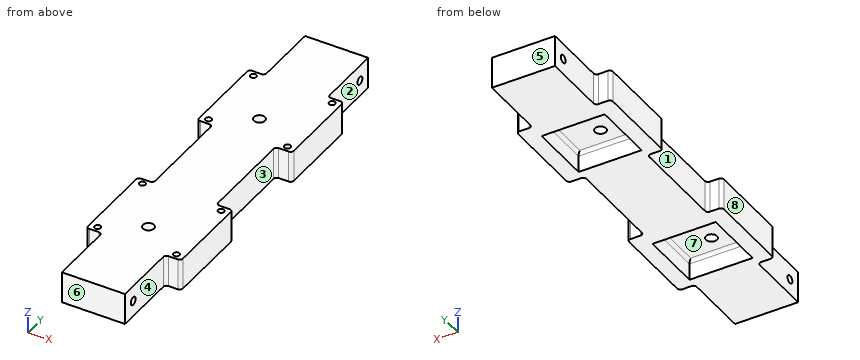
```python
from build123d import *

# Parameters (mm, degrees)
SKETCH1_W                        = 69.85
SKETCH1_H                        = 76.2
SKETCH1_R                        = 4.445
BOSS_EXTRUDE1_DEPTH              = 25.4
SKETCH2_W                        = 50.8
SKETCH2_H                        = 49.911
CUT_EXTRUDE1_DEPTH               = 15.875
SKETCH4_W                        = 50.8
SKETCH4_H                        = 25.4
BOSS_EXTRUDE2_DEPTH              = 79.9846
SKETCH7_W                        = 76.2
SKETCH7_H                        = 25.4
BOSS_EXTRUDE5_DEPTH              = 69.85
SKETCH10_R                       = 4.445
CUT_EXTRUDE3_DEPTH               = 191.349362468
SKETCH11_W                       = 50.8
SKETCH11_H                       = 49.911
CUT_EXTRUDE4_DEPTH               = 15.875
SKETCH12_W                       = 50.8
SKETCH12_H                       = 25.4
BOSS_EXTRUDE7_DEPTH              = 54.4576
SKETCH13_W                       = 50.8
SKETCH13_H                       = 25.4
BOSS_EXTRUDE8_DEPTH              = 54.2798
F_10_0_1935_DIAMETER_HOLE2_D     = 4.9149
F_10_0_1935_DIAMETER_HOLE2_DEPTH = 11.938
F_10_0_1935_DIAMETER_HOLE2_TIP   = 1.476584928
SKETCH18_R                       = 3.2639
CUT_EXTRUDE5_DEPTH               = 12.7
CUT_EXTRUDE6_START               = -12.7
SKETCH19_R                       = 3.2639
CUT_EXTRUDE6_DEPTH               = 12.7
SKETCH20_R                       = 3.2639
CUT_EXTRUDE7_DEPTH               = 12.7
CUT_EXTRUDE8_START               = -12.7
SKETCH21_R                       = 3.2639
CUT_EXTRUDE8_DEPTH               = 12.7
F_10_0_1935_DIAMETER_HOLE3_D     = 4.9149
F_10_0_1935_DIAMETER_HOLE3_DEPTH = 11.938
F_10_0_1935_DIAMETER_HOLE3_TIP   = 1.476584928
FILLET1_R                        = 2.54
FILLET2_R                        = 2.54


with BuildPart() as part:
    # Sketch1 → Boss-Extrude1 (new body)
    with BuildSketch(Plane(origin=(0, 0, 0), x_dir=(0, 1, 0), z_dir=(0, 0, 1))):
        Rectangle(SKETCH1_W, SKETCH1_H)
        with Locations(Location((-11.811, 1.778, 0), (0, 0, 270))):
            Circle(SKETCH1_R, mode=Mode.SUBTRACT)
    extrude(amount=BOSS_EXTRUDE1_DEPTH)

    # Sketch2 → Cut-Extrude1 (cut)
    with BuildSketch(Plane(origin=(0, 0, 0), x_dir=(1, 0, 0), z_dir=(0, 0, -1))):
        with Locations((0, 2.7305)):
            Rectangle(SKETCH2_W, SKETCH2_H)
    extrude(amount=-CUT_EXTRUDE1_DEPTH, mode=Mode.SUBTRACT)

    # Sketch4 → Boss-Extrude2 (add)
    with BuildSketch(Plane(origin=(0, 34.925, 0), x_dir=(-1, 0, 0), z_dir=(0, 1, 0))):
        with Locations((0.465931196, 12.7)):
            Rectangle(SKETCH4_W, SKETCH4_H)
    extrude(amount=BOSS_EXTRUDE2_DEPTH)

    # Sketch7 → Boss-Extrude5 (add)
    with BuildSketch(Plane(origin=(0, 114.9096, 0), x_dir=(-1, 0, 0), z_dir=(0, 1, 0))):
        with Locations((0, 12.7)):
            Rectangle(SKETCH7_W, SKETCH7_H)
    extrude(amount=BOSS_EXTRUDE5_DEPTH)

    # Sketch10 → Cut-Extrude3 (cut, through all)
    with BuildSketch(Plane.XY.offset(25.4)):
        with Locations((-1.778, 138.0236)):
            Circle(SKETCH10_R)
    extrude(amount=-CUT_EXTRUDE3_DEPTH, mode=Mode.SUBTRACT)

    # Sketch11 → Cut-Extrude4 (cut)
    with BuildSketch(Plane(origin=(0, 0, 0), x_dir=(1, 0, 0), z_dir=(0, 0, -1))):
        with Locations((0, -147.1041)):
            Rectangle(SKETCH11_W, SKETCH11_H)
    extrude(amount=-CUT_EXTRUDE4_DEPTH, mode=Mode.SUBTRACT)

    # Sketch12 → Boss-Extrude7 (add)
    with BuildSketch(Plane(origin=(0, 184.7596, 0), x_dir=(-1, 0, 0), z_dir=(0, 1, 0))):
        with Locations((0, 12.7)):
            Rectangle(SKETCH12_W, SKETCH12_H)
    extrude(amount=BOSS_EXTRUDE7_DEPTH)

    # Sketch13 → Boss-Extrude8 (add)
    with BuildSketch(Plane.XZ.offset(34.925)):
        with Locations((0, 12.7)):
            Rectangle(SKETCH13_W, SKETCH13_H)
    extrude(amount=BOSS_EXTRUDE8_DEPTH)

    # #10 (0.1935) Diameter Hole2
    with Locations(Plane.XY.offset(25.4)):
        with Locations((31.75, 119.6721), (31.75, 179.9971), (-31.75, 179.9971), (-31.75, 119.6721)):
            Hole(F_10_0_1935_DIAMETER_HOLE2_D / 2, depth=F_10_0_1935_DIAMETER_HOLE2_DEPTH)
            with Locations((0, 0, -(F_10_0_1935_DIAMETER_HOLE2_DEPTH + F_10_0_1935_DIAMETER_HOLE2_TIP / 2))):  # 118° drill point
                Cone(0, F_10_0_1935_DIAMETER_HOLE2_D / 2, F_10_0_1935_DIAMETER_HOLE2_TIP, mode=Mode.SUBTRACT)

    # Sketch18 → Cut-Extrude5 (cut)
    with BuildSketch(Plane.YZ.offset(25.4)):
        with Locations(Location((228.1047, 12.7, 0), (0, 0, 270))):
            Circle(SKETCH18_R)
    extrude(amount=-CUT_EXTRUDE5_DEPTH, mode=Mode.SUBTRACT)

    # Sketch19 → Cut-Extrude6 (cut)
    with BuildSketch(Plane(origin=(-25.4, 0, 0), x_dir=(0, -1, 0), z_dir=(-1, 0, 0)).offset(CUT_EXTRUDE6_START)):
        with Locations(Location((-228.1047, 12.7, 0), (0, 0, 270))):
            Circle(SKETCH19_R)
    extrude(amount=CUT_EXTRUDE6_DEPTH, mode=Mode.SUBTRACT)

    # Sketch20 → Cut-Extrude7 (cut)
    with BuildSketch(Plane(origin=(-25.4, 0, 0), x_dir=(0, -1, 0), z_dir=(-1, 0, 0))):
        with Locations(Location((78.0923, 12.7, 0), (0, 0, 90))):
            Circle(SKETCH20_R)
    extrude(amount=-CUT_EXTRUDE7_DEPTH, mode=Mode.SUBTRACT)

    # Sketch21 → Cut-Extrude8 (cut)
    with BuildSketch(Plane.YZ.offset(25.4).offset(CUT_EXTRUDE8_START)):
        with Locations(Location((-78.0923, 12.7, 0), (0, 0, 90))):
            Circle(SKETCH21_R)
    extrude(amount=CUT_EXTRUDE8_DEPTH, mode=Mode.SUBTRACT)

    # #10 (0.1935) Diameter Hole3
    with Locations(Plane.XY.offset(25.4)):
        with Locations((31.75, -30.1625), (31.663484949, 30.1625), (-31.75, 30.1625), (-31.75, -30.1625)):
            Hole(F_10_0_1935_DIAMETER_HOLE3_D / 2, depth=F_10_0_1935_DIAMETER_HOLE3_DEPTH)
            with Locations((0, 0, -(F_10_0_1935_DIAMETER_HOLE3_DEPTH + F_10_0_1935_DIAMETER_HOLE3_TIP / 2))):  # 118° drill point
                Cone(0, F_10_0_1935_DIAMETER_HOLE3_D / 2, F_10_0_1935_DIAMETER_HOLE3_TIP, mode=Mode.SUBTRACT)

    # Fillet1
    fillet1_edges = [part.edges().sort_by_distance(p)[0] for p in [
        (-25.4, -34.925, 12.7),
        (25.4, -34.925, 12.7),
        (24.934068804, 34.925, 12.7),
        (-25.865931196, 34.925, 12.7),
        (24.934068804, 114.9096, 12.7),
        (-25.865931196, 114.9096, 12.7),
        (38.1, 114.9096, 12.7),
        (-38.1, 114.9096, 12.7),
        (38.1, 184.7596, 12.7),
        (-38.1, 184.7596, 12.7),
        (38.1, 34.925, 12.7),
        (38.1, -34.925, 12.7),
        (-38.1, -34.925, 12.7),
        (-38.1, 34.925, 12.7),
        (25.4, 184.7596, 12.7),
        (-25.4, 184.7596, 12.7),
    ]]
    fillet(fillet1_edges, radius=FILLET1_R)

    # Fillet2
    fillet2_edges = [part.edges().sort_by_distance(p)[0] for p in [
        (-25.4, -2.7305, 15.875),
        (0, -27.686, 15.875),
        (25.4, -2.7305, 15.875),
        (0, 22.225, 15.875),
        (-25.4, 147.1041, 15.875),
        (0, 122.1486, 15.875),
        (25.4, 147.1041, 15.875),
        (0, 172.0596, 15.875),
    ]]
    fillet(fillet2_edges, radius=FILLET2_R)


solid = part.part
```
Model file for the job. Use its own axes, mm. Face numbers are marked on the shaded views. A direction names the side the tool comes from. Round coordinates to 2 decimals unless told otherwise and drop trailing zeros. Loops run counter-clockwise (first coordinate to the right, second up) from the corner with the lowest first, then second, coordinate; pieces in that order, holes last. Notation, with made-up numbers: M 13,61 L 39,61 A30 ccw 39,86 Z; hole C 58.5,11 d2. An arc over 180 degrees is marked long. Put each result on its own line as item: value. Start each with the question number.
Item 1: Mould opens along Y. For the marked faces 5, 6, 7 and 8 say: released by +Y, released by -Y, zero draft, split by the parting line, or undercut.
Item 2: Cut at A-A (y = 6). List the corners of the cut face in (x, z) (3 decimals), then the cut area to 3 significant figures.
Item 3: Drop flat-ended pins along their axis: P1, Ø10, axis at x = -1.78, y = 138.02, coming from the -Z side (3 decimals); P2, Ø2, axis at y = -77, z = 11.5, coming from the +X side; P3, Ø6, axis at x = 33, z = 7.5, coming from the -Y side (3 decimals). Give the stop position or say it passes through.
Item 4: Cut at C-C (y = 46.5). List the corners of the cut face in (x, z).
Item 5: Cut at B-B (x = -18). List the corners of the cut face in (y, z) (3 decimals), then the cut area to 3 significant figures.
Item 6: 3-axis set-ups, long thin cutter, end or side, ignore diameter. For the marked faces 1, 2, 3 and 4: which of +Z, -Z, +X, -X, +Y, -Y reach the whole face in a straight line?
Item 7: Drill centre lines: line 1 along Y through (x, z) = (-31.75, 17.5) (3 decimals); line 2 along Y through (x, z) = (4, 6.75) (3 decimals); line 3 along Y through (x, z) = (17, 12.7) (3 decimals). Where is each one in solid material? Low to high.
Answer block:
1. face 5: released by +Y
1. face 6: released by -Y
1. face 7: undercut
1. face 8: zero draft
2. outline: M -38.1,0 L -25.4,0 L -25.4,13.335 A2.54 cw -22.86,15.875 L 22.86,15.875 A2.54 cw 25.4,13.335 L 25.4,0 L 38.1,0 L 38.1,25.4 L -38.1,25.4 Z
2. area: 1,130 mm2
3. P1: z = 15.875
3. P2: x = 12.7
3. P3: y = -34.925
4. outline: M -25.87,0 L 24.93,0 L 24.93,25.4 L -25.87,25.4 Z
5. outline: M -89.205,0 L -27.686,0 L -27.686,13.335 A2.54 cw -25.146,15.875 L 19.685,15.875 A2.54 cw 22.225,13.335 L 22.225,0 L 122.149,0 L 122.149,13.335 A2.54 cw 124.689,15.875 L 169.52,15.875 A2.54 cw 172.06,13.335 L 172.06,0 L 239.217,0 L 239.217,25.4 L -89.205,25.4 Z; hole C -78.092,12.7 d6.528; hole C 228.105,12.7 d6.528
5. area: 6,700 mm2
6. face 1: +Z, -Z, -X
6. face 2: +Z, -Z, +X, +Y
6. face 3: +Z, -Z, +X
6. face 4: +Z, -Z, +X, -Y
7. line 1: -34.925 to -32.62, -27.705 to 27.705, 32.62 to 34.925, 114.91 to 117.215, 122.13 to 177.54, 182.455 to 184.76
7. line 2: -89.205 to -27.686, 22.225 to 122.149, 172.06 to 239.217
7. line 3: -89.205 to -81.356, -74.828 to -27.686, 22.225 to 122.149, 172.06 to 224.841, 231.369 to 239.217
